Can you work these out from the model? Positions are in its coordinate system, mm. A direction names the side the tool comes from. Round coordinates to 2 decimals unless told otherwise and drop trailing zeros. Loops run counter-clockwise (first coordinate to the right, second up) from the corner with the lowest first, then second, coordinate; pieces in that order, holes last. Notation, with made-up numbers: (71, 61) - (124, 61) arc R28 ccw to (124, 91) - close; hole circle Ø8 at (86.25, 37). An arc over 180 degrees is marked (long way). Answer as CSV lines item,"result".
```python
from build123d import *

# Parameters (mm, degrees)
SKETCH_W        = 70
SKETCH_H        = 70
PAD_DEPTH       = 2
PAD001_DEPTH    = 22
POCKET_DEPTH    = 22
SKETCH003_W     = 16
SKETCH003_H     = 23.864653
POCKET001_DEPTH = 18
SKETCH005_W     = 41.4
SKETCH005_H     = 15.4
PAD003_DEPTH    = 4
SKETCH006_W     = 39
SKETCH006_H     = 13
POCKET002_DEPTH = 5
SKETCH007_W     = 23
SKETCH007_H     = 7
POCKET003_DEPTH = 1.001
POCKET004_DEPTH = 5
SKETCH009_R     = 1.6
POCKET005_DEPTH = 58.501
SKETCH010_R     = 2
SKETCH010_W     = 2.5
SKETCH010_H     = 3
SKETCH010_W_2   = 3
PAD004_DEPTH    = 7
POCKET006_DEPTH = 5
POCKET007_DEPTH = 2
FILLET_R        = 15
SKETCH014_W     = 3
SKETCH014_H     = 4
POCKET009_DEPTH = 4
SKETCH015_R     = 1
POCKET010_DEPTH = 24.001


with BuildPart() as part:
    # Sketch → Pad (new body)
    with BuildSketch(Plane.XY):
        Rectangle(SKETCH_W, SKETCH_H)
        with BuildLine():
            ThreePointArc((27.608372, -4.666667), (28, 0), (27.608372, 4.666667))
            ThreePointArc((31.552426, 5.333333), (29.247066, 6.972027), (27.608372, 4.666667))
            ThreePointArc((31.552426, -5.333333), (32, 0), (31.552426, 5.333333))
            ThreePointArc((27.608372, -4.666667), (29.247066, -6.972027), (31.552426, -5.333333))
        make_face(mode=Mode.SUBTRACT)
        with BuildLine():
            ThreePointArc((-27.608372, 4.666667), (-28, 0), (-27.608372, -4.666667))
            ThreePointArc((-31.552426, -5.333333), (-29.247066, -6.972027), (-27.608372, -4.666667))
            ThreePointArc((-31.552426, 5.333333), (-32, 0), (-31.552426, -5.333333))
            ThreePointArc((-27.608372, 4.666667), (-29.247066, 6.972027), (-31.552426, 5.333333))
        make_face(mode=Mode.SUBTRACT)
        with BuildLine():
            ThreePointArc((4.666667, 27.608372), (-1e-06, 28), (-4.666668, 27.608372))
            ThreePointArc((-5.333333, 31.552426), (-6.972027, 29.247066), (-4.666668, 27.608372))
            ThreePointArc((5.333333, 31.552426), (0, 32), (-5.333333, 31.552426))
            ThreePointArc((4.666667, 27.608372), (6.972027, 29.247066), (5.333333, 31.552426))
        make_face(mode=Mode.SUBTRACT)
        with BuildLine():
            ThreePointArc((-4.666659, -27.608374), (4e-06, -28), (4.666667, -27.608372))
            ThreePointArc((5.333333, -31.552426), (6.972027, -29.247066), (4.666667, -27.608372))
            ThreePointArc((-5.333319, -31.552428), (7e-06, -32), (5.333333, -31.552426))
            ThreePointArc((-4.666659, -27.608374), (-6.972027, -29.247069), (-5.333319, -31.552428))
        make_face(mode=Mode.SUBTRACT)
    extrude(amount=PAD_DEPTH)

    # Sketch001 (on Face22 of Pad) → Pad001 (join)
    with BuildSketch(Plane.XY.offset(2)):
        with BuildLine():
            Line((21.719807, -23.5), (-21.719807, -23.5))
            ThreePointArc((-23.5, -21.719807), (-22.627417, -22.627417), (-21.719807, -23.5))
            Line((-23.5, 21.719807), (-23.5, -21.719807))
            ThreePointArc((-21.719807, 23.5), (-22.627417, 22.627417), (-23.5, 21.719807))
            Line((-21.719807, 23.5), (21.719807, 23.5))
            ThreePointArc((23.5, 21.719807), (22.627417, 22.627417), (21.719807, 23.5))
            Line((23.5, 21.719807), (23.5, -21.719807))
            ThreePointArc((21.719807, -23.5), (22.627417, -22.627417), (23.5, -21.719807))
        make_face()
    extrude(amount=PAD001_DEPTH)

    # Sketch002 (on Face31 of Pad001) → Pocket (cut)
    with BuildSketch(Plane.XY.offset(24)):
        with BuildLine():
            Line((-22.3, 21.244999), (-22.3, -21.244999))
            ThreePointArc((-22.3, -21.244999), (-21.778889, -21.778889), (-21.244999, -22.3))
            Line((-21.244999, -22.3), (21.244999, -22.3))
            ThreePointArc((21.244999, -22.3), (21.778889, -21.778889), (22.3, -21.244999))
            Line((22.3, 21.244999), (22.3, -21.244999))
            ThreePointArc((22.3, 21.244999), (21.778889, 21.778889), (21.244999, 22.3))
            Line((-21.244999, 22.3), (21.244999, 22.3))
            ThreePointArc((-21.244999, 22.3), (-21.778889, 21.778889), (-22.3, 21.244999))
        make_face()
    extrude(amount=-POCKET_DEPTH, mode=Mode.SUBTRACT)

    # Sketch003 (on Face23 of Pocket) → Pocket001 (cut)
    with BuildSketch(Plane.XZ.offset(23.5)):
        with Locations((12.5, 21.932326)):
            Rectangle(SKETCH003_W, SKETCH003_H)
    extrude(amount=-POCKET001_DEPTH, mode=Mode.SUBTRACT)

    # Sketch005 (on Face43 of Pocket001) → Pad003 (join)
    with BuildSketch(Plane.XY.offset(2)):
        with Locations((0, -12)):
            Rectangle(SKETCH005_W, SKETCH005_H)
    extrude(amount=PAD003_DEPTH)

    # Sketch006 (on Face48 of Pad003) → Pocket002 (cut)
    with BuildSketch(Plane.XY.offset(6)):
        with Locations((0, -12)):
            Rectangle(SKETCH006_W, SKETCH006_H)
    extrude(amount=-POCKET002_DEPTH, mode=Mode.SUBTRACT)

    # Sketch007 (on Face53 of Pocket002) → Pocket003 (cut, through all)
    with BuildSketch(Plane.XY.offset(1)):
        with Locations((0, -11)):
            Rectangle(SKETCH007_W, SKETCH007_H)
    extrude(amount=-POCKET003_DEPTH, mode=Mode.SUBTRACT)

    # Sketch008 (on Face53 of Pocket003) → Pocket004 (cut)
    with BuildSketch(Plane.XY.offset(2)):
        with BuildLine():
            Line((-20.25, 17.174446), (-20.25, 0.174446))
            ThreePointArc((-20.25, 0.174446), (-18.25, -1.825554), (-16.25, 0.174446))
            Line((-16.25, 17.174446), (-16.25, 0.174446))
            ThreePointArc((-16.25, 17.174446), (-18.25, 19.174446), (-20.25, 17.174446))
        make_face()
        with BuildLine():
            Line((-12.95, 17.174446), (-12.95, 0.174446))
            ThreePointArc((-12.95, 0.174446), (-10.95, -1.825554), (-8.95, 0.174446))
            Line((-8.95, 17.174446), (-8.95, 0.174446))
            ThreePointArc((-8.95, 17.174446), (-10.95, 19.174446), (-12.95, 17.174446))
        make_face()
        with BuildLine():
            Line((-5.65, 17.174446), (-5.65, 0.174446))
            ThreePointArc((-5.65, 0.174446), (-3.65, -1.825554), (-1.65, 0.174446))
            Line((-1.65, 17.174446), (-1.65, 0.174446))
            ThreePointArc((-1.65, 17.174446), (-3.65, 19.174446), (-5.65, 17.174446))
        make_face()
        with BuildLine():
            Line((1.65, 17.174446), (1.65, 0.174446))
            ThreePointArc((1.65, 0.174446), (3.65, -1.825554), (5.65, 0.174446))
            Line((5.65, 17.174446), (5.65, 0.174446))
            ThreePointArc((5.65, 17.174446), (3.65, 19.174446), (1.65, 17.174446))
        make_face()
        with BuildLine():
            Line((8.95, 17.174446), (8.95, 0.174446))
            ThreePointArc((8.95, 0.174446), (10.95, -1.825554), (12.95, 0.174446))
            Line((12.95, 17.174446), (12.95, 0.174446))
            ThreePointArc((12.95, 17.174446), (10.95, 19.174446), (8.95, 17.174446))
        make_face()
        with BuildLine():
            Line((16.25, 17.174446), (16.25, 0.174446))
            ThreePointArc((16.25, 0.174446), (18.25, -1.825554), (20.25, 0.174446))
            Line((20.25, 17.174446), (20.25, 0.174446))
            ThreePointArc((20.25, 17.174446), (18.25, 19.174446), (16.25, 17.174446))
        make_face()
        with BuildLine():
            Line((3.5, -20.045416), (17.5, -20.045416))
            ThreePointArc((17.5, -22.045416), (18.5, -21.045416), (17.5, -20.045416))
            Line((3.5, -22.045416), (17.5, -22.045416))
            ThreePointArc((3.5, -20.045416), (2.5, -21.045416), (3.5, -22.045416))
        make_face()
        with BuildLine():
            Line((-17.5, -20.045416), (-3.5, -20.045416))
            ThreePointArc((-3.5, -22.045416), (-2.5, -21.045416), (-3.5, -20.045416))
            Line((-17.5, -22.045416), (-3.5, -22.045416))
            ThreePointArc((-17.5, -20.045416), (-18.5, -21.045416), (-17.5, -22.045416))
        make_face()
    extrude(amount=-POCKET004_DEPTH, mode=Mode.SUBTRACT)

    # Sketch009 (on Face59 of Pocket004) → Pocket005 (cut, through all)
    with BuildSketch(Plane.XZ.offset(23.5)):
        with Locations((0, 20)):
            Circle(SKETCH009_R)
    extrude(amount=-POCKET005_DEPTH, mode=Mode.SUBTRACT)

    # Sketch010 (on Face67 of Pocket005) → Pad004 (join)
    with BuildSketch(Plane.XY.offset(2)):
        with Locations((21, 21)):
            Circle(SKETCH010_R)
        with Locations((-21, 21)):
            Circle(SKETCH010_R)
        with Locations((-21, -21)):
            Circle(SKETCH010_R)
        with Locations((21.75, 4.5)):
            Rectangle(SKETCH010_W, SKETCH010_H)
        with Locations((0, -21)):
            Rectangle(SKETCH010_W_2, SKETCH010_H)
    extrude(amount=PAD004_DEPTH)

    # Sketch011 (on Face63 of Pad004) → Pocket006 (cut)
    with BuildSketch(Plane(origin=(0, 23.5, 0), x_dir=(-1, 0, 0), z_dir=(0, 1, 0))):
        with BuildLine():
            Line((-18.5, 17.993099), (-18.5, 5.993099))
            ThreePointArc((-18.5, 5.993099), (-16.5, 3.993099), (-14.5, 5.993099))
            Line((-14.5, 17.993099), (-14.5, 5.993099))
            ThreePointArc((-14.5, 17.993099), (-16.5, 19.993099), (-18.5, 17.993099))
        make_face()
        with BuildLine():
            Line((-7.5, 17.993099), (-7.5, 5.993099))
            ThreePointArc((-7.5, 5.993099), (-5.5, 3.993099), (-3.5, 5.993099))
            Line((-3.5, 17.993099), (-3.5, 5.993099))
            ThreePointArc((-3.5, 17.993099), (-5.5, 19.993099), (-7.5, 17.993099))
        make_face()
        with BuildLine():
            Line((3.5, 17.993099), (3.5, 5.993099))
            ThreePointArc((3.5, 5.993099), (5.5, 3.993099), (7.5, 5.993099))
            Line((7.5, 17.993099), (7.5, 5.993099))
            ThreePointArc((7.5, 17.993099), (5.5, 19.993099), (3.5, 17.993099))
        make_face()
        with BuildLine():
            Line((14.5, 17.993099), (14.5, 5.993099))
            ThreePointArc((14.5, 5.993099), (16.5, 3.993099), (18.5, 5.993099))
            Line((18.5, 17.993099), (18.5, 5.993099))
            ThreePointArc((18.5, 17.993099), (16.5, 19.993099), (14.5, 17.993099))
        make_face()
    extrude(amount=-POCKET006_DEPTH, mode=Mode.SUBTRACT)

    # Sketch012 (on Face59 of Pocket006) → Pocket007 (cut)
    with BuildSketch(Plane.XZ.offset(23.5)):
        with BuildLine():
            Line((-17, 18), (-17, 6))
            ThreePointArc((-17, 6), (-15, 4), (-13, 6))
            Line((-13, 18), (-13, 6))
            ThreePointArc((-13, 18), (-15, 20), (-17, 18))
        make_face()
        with BuildLine():
            Line((-6, 18), (-6, 6))
            ThreePointArc((-6, 6), (-4, 4), (-2, 6))
            Line((-2, 18), (-2, 6))
            ThreePointArc((-2, 18), (-4, 20), (-6, 18))
        make_face()
    extrude(amount=-POCKET007_DEPTH, mode=Mode.SUBTRACT)

    # Fillet
    fillet_edges = [part.edges().sort_by_distance(p)[0] for p in [
        (-35, -35, 1),
        (-35, 35, 1),
        (35, -35, 1),
        (35, 35, 1),
    ]]
    fillet(fillet_edges, radius=FILLET_R)

    # Sketch014 (on Face2 of Fillet) → Pocket009 (cut)
    with BuildSketch(Plane(origin=(0, 0, 0), x_dir=(1, 0, 0), z_dir=(0, 0, -1))):
        with Locations((-23.5, -11)):
            Rectangle(SKETCH014_W, SKETCH014_H)
    extrude(amount=-POCKET009_DEPTH, mode=Mode.SUBTRACT)

    # Sketch015 (on Face2 of Pocket009) → Pocket010 (cut, through all)
    with BuildSketch(Plane(origin=(0, 0, 0), x_dir=(1, 0, 0), z_dir=(0, 0, -1))):
        with Locations((-21, 21)):
            Circle(SKETCH015_R)
        with Locations((-21, -21)):
            Circle(SKETCH015_R)
    extrude(amount=-POCKET010_DEPTH, mode=Mode.SUBTRACT)


solid = part.part
```
Q1. I'm going to push flat-ended pins straight in: pin 1 Ø2 at (y, z) = (-14.5, 4) entering from -X; pin 2 Ø11 at (y, z) = (9.5, 10.5) entering from +X; pin 3 Ø6.5 at (x, y) = (5, -10.5) entering from +Z. Where does each tip first touch, or does it pass through?
Checks:
pin 1,"x = -23.5"
pin 2,"x = 23.5"
pin 3,"z = 1"
Q2. Imagine slicing it at B-B (z = 12.75). Count the separate pieces of the cut face and the enclosed holes in it, then the cut area to 3 significant figures.
Checks:
separate pieces,"7"
enclosed holes,"0"
area,"168 mm²"
Q3. We'd pull the mould along Y, two halves only. Please class faces 4 (the cylindrical face through (-5.456, 22.908, 3.994)), 5 (the cylindrical face through (-22.64, -22.615, 12.846)), 6 (the cylindrical face through (-22.615, 22.64, 12.846)), 7 (the flat face through (-19.5, -12, 4)): pulls with the +Y half, pulls with the -Y half, needs draft (parallel to the pull), parting line crosses it, or undercut.
Checks:
face 4,"needs draft"
face 5,"pulls with the -Y half"
face 6,"pulls with the +Y half"
face 7,"undercut"
Q4. Imagine slicing it at A-A (y = -9). Write out the boundary of the cut face in (x, z).
Checks:
outline,"(-35, 0) - (-11.5, 0) - (-11.5, 1) - (-19.5, 1) - (-19.5, 6) - (-20.7, 6) - (-20.7, 2) - (-22.3, 2) - (-22.3, 24) - (-23.5, 24) - (-23.5, 2) - (-35, 2) - close; (11.5, 0) - (35, 0) - (35, 2) - (23.5, 2) - (23.5, 24) - (22.3, 24) - (22.3, 2) - (20.7, 2) - (20.7, 6) - (19.5, 6) - (19.5, 1) - (11.5, 1) - close"
Q5. Imagine slicing it at D-D (x = 25). Write out the boundary of the cut face in (y, z), then the cut area to 3 significant figures.
Checks:
outline,"(-34.14, 0) - (34.14, 0) - (34.14, 2) - (-34.14, 2) - close"
area,"137 mm²"
Q6. On a 3-axis mill with a long thin cutter (end or side, diameter ignored), from which of +Z, -Z, +X, -X, +Y, -Y can I reach the whole of each face in a straight line? I mean faces 1 (the flat face through (-23.5, 0, 13)), 2 (the cylindrical face through (-15, -23, 20)), 3 (the flat face through (-23.5, 13, 1.5)). Say none if no direction works.
Checks:
face 1,"+Z, -X, +Y, -Y"
face 2,"-Y"
face 3,"-Z"
Q7. If I drill on line 1 along X through (y, z) = (-21, 4.5); line 2 along Y through (x, z) = (-21, 4); line 3 along X through (y, z) = (21, 2.25), over which ranges is the centre line in solid material (lowest first)? Write a range as [from, to].
Checks:
line 1,"[-23.5, -22], [-20, -19], [-1.5, 1.5], [22.3, 23.5]"
line 2,"[-23.5, -22], [-20, -19], [19, 20], [22, 23.5]"
line 3,"[-23.5, -22], [-20, -19], [19, 23.5]"
